Work out the finished part from the listing and answer in its coordinate system (mm). Face numbers are marked on the shaded views. A direction names the side the tool comes from. Coordinates: 2 decimals unless noted, no trailing zeros. Loops run counter-clockwise (first coordinate to the right, second up) from the corner with the lowest first, then second, coordinate; pieces in that order, holes last. Notation, with made-up numbers: (25, 56.5) -> (83, 56.5) arc R35 cw to (83, 88.5) -> close; hole circle Ø2 at (81.5, -21.5). An arc over 180 degrees is marked (long way). Use a Markdown table: item, result.
from build123d import *

# Parameters (mm, degrees)
SKETCH_1_R          = 2.75
EXTRUDE_1_DEPTH     = 3
FILLET_1_R          = 0.5
CUT_EXTRUDE_1_DEPTH = 2
SKETCH_3_R          = 1.5
EXTRUDE_2_DEPTH     = 10
CHAMFER_1_SIZE      = 0.2
FILLET_2_R          = 0.2


with BuildPart() as part:
    # 草图1 → 凸台-拉伸1 (new body)
    with BuildSketch(Plane.XY):
        Circle(SKETCH_1_R)
    extrude(amount=EXTRUDE_1_DEPTH)

    # 圆角1
    fillet_1_edges = [part.edges().sort_by_distance(p)[0] for p in [
        (-2.75, 0, 3),
    ]]
    fillet(fillet_1_edges, radius=FILLET_1_R)

    # 草图2 → 切除-拉伸1 (cut)
    with BuildSketch(Plane.XY.offset(3)):
        Polygon((1.558845727, 0), (0.779422863, 1.35), (-0.779422863, 1.35), (-1.558845727, 0), (-0.779422863, -1.35), (0.779422863, -1.35), align=None)
    extrude(amount=-CUT_EXTRUDE_1_DEPTH, mode=Mode.SUBTRACT)

    # 草图3 → 凸台-拉伸2 (add)
    with BuildSketch(Plane(origin=(0, 0, 0), x_dir=(-1, 0, 0), z_dir=(0, 0, -1))):
        Circle(SKETCH_3_R)
    extrude(amount=EXTRUDE_2_DEPTH)

    # 倒角1
    chamfer_1_edges = [part.edges().sort_by_distance(p)[0] for p in [
        (1.5, 0, -10),
    ]]
    chamfer(chamfer_1_edges, length=CHAMFER_1_SIZE)

    # 圆角2
    fillet_2_edges = [part.edges().sort_by_distance(p)[0] for p in [
        (-2.75, 0, 0),
    ]]
    fillet(fillet_2_edges, radius=FILLET_2_R)


solid = part.part
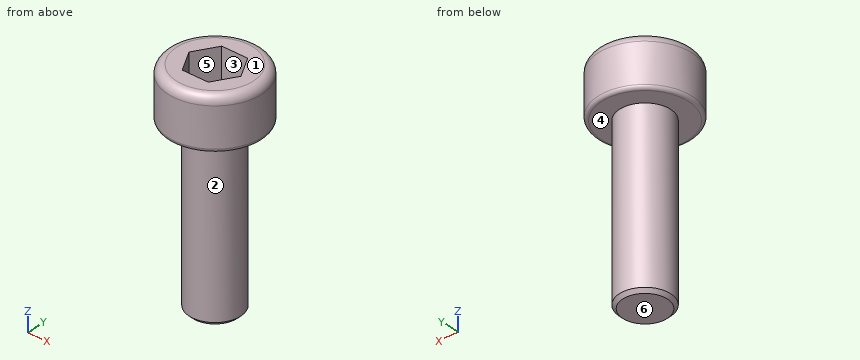
Q1. For the marked faces 4, 5 and 6, determine the directions among +Z, -Z, +X, -X, +Y, -Y from which every point of the face is accessible in a straight line to the end or side of a thin tool.
Solved:
| item | result |
|---|---|
| face 4 | -Z |
| face 5 | +Z |
| face 6 | -Z, +X, -X, +Y, -Y |
Q2. Consider line 1 (X direction, y = 0.1, z = 0.5); line 2 (Z direction, x = -1.6, y = 1.2); line 3 (X direction, y = 0.1, z = -3.5). Determine where each line is inside the solid, lowest interval first. Write a range as [from, to].
Solved:
| item | result |
|---|---|
| line 1 | [-2.75, 2.75] |
| line 2 | [0, 3] |
| line 3 | [-1.5, 1.5] |
Q3. Section B-B on x = 0 is taken. Determine the outline of the cut face in (y, z), and give its area (3 significant figures).
Solved:
| item | result |
|---|---|
| outline | (-2.75, 0.2) arc R0.2 ccw to (-2.55, 0) -> (-1.5, 0) -> (-1.5, -9.8) -> (-1.3, -10) -> (1.3, -10) -> (1.5, -9.8) -> (1.5, 0) -> (2.55, 0) arc R0.2 ccw to (2.75, 0.2) -> (2.75, 2.5) arc R0.5 ccw to (2.25, 3) -> (1.35, 3) -> (1.35, 1) -> (-1.35, 1) -> (-1.35, 3) -> (-2.25, 3) arc R0.5 ccw to (-2.75, 2.5) -> close |
| area | 40.9 mm² |
Q4. Section C-C on z = 0.5 is taken. Determine the outline of the cut face in (x, y), and give its area (3 significant figures).
Solved:
| item | result |
|---|---|
| outline | circle Ø5.5 at (0, 0) |
| area | 23.8 mm² |
Q5. Given pin 1 Ø3 at (y, z) = (2, -7.5) entering from +X; pin 2 Ø1.5 at (x, y) = (-1.5, -2) entering from -Z; pin 3 Ø0.8 at (x, z) = (-0.5, 2) entering from +Y, each flat-ended and moving along its own axis, determine where each tip first touches the part or whether it passes through.
Solved:
| item | result |
|---|---|
| pin 1 | x = 1.41 |
| pin 2 | z = 0 |
| pin 3 | y = 2.75 |
Q6. Determine the mould class of the marked faces 1, 2 and 3 for opening direction X: pulls with the +X half, pulls with the -X half, needs draft (parallel to the pull), parting line crosses it, or undercut.
Solved:
| item | result |
|---|---|
| face 1 | needs draft |
| face 2 | parting line crosses it |
| face 3 | undercut |
Q7. Section D-D on z = -2.25 is taken. Determine the outline of the cut face in (x, y).
Solved:
| item | result |
|---|---|
| outline | circle Ø3 at (0, 0) |
Q8. Section A-A on z = 2.25 is taken. Determine the outline of the cut face in (x, y), and give its area (3 significant figures).
Solved:
| item | result |
|---|---|
| outline | circle Ø5.5 at (0, 0); hole (-1.56, 0) -> (-0.78, -1.35) -> (0.78, -1.35) -> (1.56, 0) -> (0.78, 1.35) -> (-0.78, 1.35) -> close |
| area | 17.4 mm² |
